```python
from build123d import *

# Parameters (mm, degrees)
SKETCH1_W           = 70
SKETCH1_H           = 40
BOSS_EXTRUDE1_DEPTH = 50
SKETCH2_W           = 20
SKETCH2_H           = 30
CUT_EXTRUDE1_DEPTH  = 50
SKETCH3_W           = 10
SKETCH3_H           = 20
CUT_EXTRUDE2_DEPTH  = 50
SKETCH4_W           = 30
SKETCH4_H           = 30
BOSS_EXTRUDE2_DEPTH = 10
CUT_EXTRUDE3_DEPTH  = 56


with BuildPart() as part:
    # Sketch1 → Boss-Extrude1 (new body)
    with BuildSketch(Plane.XY):
        with Locations((35, 20)):
            Rectangle(SKETCH1_W, SKETCH1_H)
    extrude(amount=BOSS_EXTRUDE1_DEPTH)

    # Sketch2 → Cut-Extrude1 (cut)
    with BuildSketch(Plane(origin=(0, 40, 0), x_dir=(1, 0, 0), z_dir=(0, 1, 0))):
        with Locations((10, -35)):
            Rectangle(SKETCH2_W, SKETCH2_H)
    extrude(amount=-CUT_EXTRUDE1_DEPTH, mode=Mode.SUBTRACT)

    # Sketch3 → Cut-Extrude2 (cut)
    with BuildSketch(Plane.ZY.offset(-20)):
        with Locations((45, 20)):
            Rectangle(SKETCH3_W, SKETCH3_H)
    extrude(amount=-CUT_EXTRUDE2_DEPTH, mode=Mode.SUBTRACT)

    # Sketch4 → Boss-Extrude2 (add)
    with BuildSketch(Plane(origin=(0, 40, 0), x_dir=(1, 0, 0), z_dir=(0, 1, 0))):
        with Locations((55, -15)):
            Rectangle(SKETCH4_W, SKETCH4_H)
    extrude(amount=BOSS_EXTRUDE2_DEPTH)

    # Sketch5 → Cut-Extrude3 (cut)
    with BuildSketch(Plane.ZY.offset(-40)):
        Polygon((10, 50), (30, 40), (30, 50), align=None)
    extrude(amount=-CUT_EXTRUDE3_DEPTH, mode=Mode.SUBTRACT)


solid = part.part
```
CAD build for the part. Positions are in the model's coordinates, mm. A direction names the side the tool comes from. Coordinates: 2 decimals unless noted, no trailing zeros. Order: outer loops, then holes, each group sorted by start corner. A loop starts at its lowest first (then second) coordinate and runs counter-clockwise, first axis right, second up. Notation, with made-up numbers: (74, -11.75) - (112, -11.75) arc R25 ccw to (112, 25.25) - close; hole circle Ø9 at (68, 45.5). An arc over 180 degrees is marked (long way). Answer in a Markdown table with one row per item.
1. Slice it at D-D, the plane z = 8. List the corners of the cut face in (x, y).
Answer:
| item | result |
|---|---|
| outline | (0, 0) - (70, 0) - (70, 50) - (40, 50) - (40, 40) - (0, 40) - close |
2. Slice it at A-A, the plane z = 41. List the corners of the cut face in (x, y).
Answer:
| item | result |
|---|---|
| outline | (20, 0) - (70, 0) - (70, 10) - (20, 10) - close; (20, 30) - (70, 30) - (70, 40) - (20, 40) - close |
3. Slice it at C-C, the plane y = 23. List the corners of the cut face in (x, z).
Answer:
| item | result |
|---|---|
| outline | (0, 0) - (70, 0) - (70, 40) - (20, 40) - (20, 20) - (0, 20) - close |
4. Pull direction Y, two halves, no side cores. Call faces 4 (the face through (45, 30, 45)), 5 (the face through (45, 35, 50)), 6 (the face through (42, 0, 25)), 7 (the face through (35, 40, 25)): +Y half, -Y half, draft (parallel to the pull), parting line (faces both ways), or undercut.
Answer:
| item | result |
|---|---|
| face 4 | undercut |
| face 5 | draft |
| face 6 | -Y half |
| face 7 | +Y half |
5. Slice it at B-B, the plane x = 59.5. List the corners of the cut face in (y, z), then the cut area to 3 significant figures.
Answer:
| item | result |
|---|---|
| outline | (0, 0) - (50, 0) - (50, 10) - (40, 30) - (40, 50) - (30, 50) - (30, 40) - (10, 40) - (10, 50) - (0, 50) - close |
| area | 2,000 mm² |
6. 3-axis set-ups, long thin cutter, end or side, ignore diameter. For faces 1 (the face through (10, 20, 20)), 2 (the face through (45, 20, 40)), 3 (the face through (40, 44, 12)): which of +Z, -Z, +X, -X, +Y, -Y reach the whole face in a straight line?
Answer:
| item | result |
|---|---|
| face 1 | +Z, -X, +Y, -Y |
| face 2 | +Z, +X, -X |
| face 3 | +Z, -Z, -X, +Y |
7. Flat gauge pins, fed straight in: P1, Ø16, axis at x = 10, y = 15, coming from the +Z side; P2, Ø5, axis at x = 35, z = 46, coming from the +Y side; P3, Ø1.5, axis at y = 31.5, z = 24.5, coming from the -X side. Where does each tip first touch, or does it go through?
Answer:
| item | result |
|---|---|
| P1 | z = 20 |
| P2 | y = 40 |
| P3 | x = 20 |
8. Drill centre lines: L1, parallel to Y at x = 18, z = 11; L2, parallel to X at y = 5, z = 29.5; L3, parallel to Z at x = 10, y = 26.5. Where is each one in solid material? Low to high. Write a range as from..to.
Answer:
| item | result |
|---|---|
| L1 | 0..40 |
| L2 | 20..70 |
| L3 | 0..20 |
